from build123d import *

# Parameters (mm, degrees)
SKETCH1_R           = 12.5
SKETCH1_R_2         = 9
BOSS_EXTRUDE1_DEPTH = 10
BOSS_EXTRUDE2_DEPTH = 15
BOSS_EXTRUDE3_DEPTH = 7.5
BOSS_EXTRUDE4_DEPTH = 15
SKETCH3_R           = 3.25
CUT_EXTRUDE1_DEPTH  = 19
SKETCH4_R           = 22.5
CUT_EXTRUDE2_DEPTH  = 151
CUT_EXTRUDE3_DEPTH  = 5


with BuildPart() as part:
    # Sketch1 → Boss-Extrude1 (new body, symmetric)
    with BuildSketch(Plane(origin=(0, 0, 0), x_dir=(0, 0, -1), z_dir=(1, 0, 0))):
        Circle(SKETCH1_R)
        Circle(SKETCH1_R_2, mode=Mode.SUBTRACT)
    extrude(amount=BOSS_EXTRUDE1_DEPTH, both=True)



with BuildPart() as body_2:
    # Sketch1_3 → Boss-Extrude2 (new body, symmetric)
    with BuildSketch(Plane(origin=(0, 0, 0), x_dir=(0, 0, -1), z_dir=(1, 0, 0))):
        with BuildLine():
            Line((22.5, -120.4), (35, -120.4))
            Line((35, -120.4), (35, -117.4))
            Line((35, -117.4), (25.322914524, -117.4))
            ThreePointArc((25.322914524, -117.4), (0, -94.9), (-25.322914524, -117.4))
            Line((-25.322914524, -117.4), (-35, -117.4))
            Line((-35, -117.4), (-35, -120.4))
            Line((-35, -120.4), (-22.5, -120.4))
            ThreePointArc((-22.5, -120.4), (0, -97.9), (22.5, -120.4))
        make_face()
    extrude(amount=BOSS_EXTRUDE2_DEPTH, both=True)


with BuildPart() as part_1:
    add(part.part)

    add(body_2.part)  # Boss-Extrude3 merges body 2
    # Sketch1_7 → Boss-Extrude3 (add, symmetric)
    with BuildSketch(Plane(origin=(0, 0, 0), x_dir=(0, 0, -1), z_dir=(1, 0, 0))):
        with BuildLine():
            ThreePointArc((-15.952867936, -100.506382817), (0, -94.9), (15.952867936, -100.506382817))
            Line((15.952867936, -100.506382817), (8, -9.604686356))
            ThreePointArc((8, -9.604686356), (0, -12.5), (-8, -9.604686356))
            Line((-8, -9.604686356), (-15.952867936, -100.506382817))
        make_face()
    extrude(amount=BOSS_EXTRUDE3_DEPTH, both=True)

    # Sketch2 → Boss-Extrude4 (add)
    with BuildSketch(Plane(origin=(0, -117.4, 0), x_dir=(1, 0, 0), z_dir=(0, 1, 0))):
        with BuildLine():
            Line((-6, 29), (-6, 17))
            Line((-6, 17), (6, 17))
            Line((6, 17), (6, 29))
            ThreePointArc((6, 29), (0, 35), (-6, 29))
        make_face()
    boss_extrude4 = extrude(amount=BOSS_EXTRUDE4_DEPTH)

    # Sketch3 → Cut-Extrude1 (cut, through all)
    with BuildSketch(Plane(origin=(0, -102.4, 0), x_dir=(1, 0, 0), z_dir=(0, 1, 0))):
        with Locations((0, 29)):
            Circle(SKETCH3_R)
    cut_extrude1 = extrude(amount=-CUT_EXTRUDE1_DEPTH, mode=Mode.SUBTRACT)

    # Mirror1: Boss-Extrude4, Cut-Extrude1 across plane
    add(boss_extrude4.mirror(Plane.XY))
    add(cut_extrude1.mirror(Plane.XY), mode=Mode.SUBTRACT)

    # Sketch4 → Cut-Extrude2 (cut)
    with BuildSketch(Plane(origin=(15, 0, 0), x_dir=(0, 0, -1), z_dir=(1, 0, 0))):
        with Locations((0, -120.4)):
            Circle(SKETCH4_R)
    extrude(amount=-CUT_EXTRUDE2_DEPTH, mode=Mode.SUBTRACT)

    # Sketch5 → Cut-Extrude3 (cut)
    with BuildSketch(Plane(origin=(7.5, 0, 0), x_dir=(0, 0, -1), z_dir=(1, 0, 0))):
        with BuildLine():
            ThreePointArc((12.438451255, -94.757556076), (0, -91.9), (-12.438451255, -94.757556076))
            Line((-12.438451255, -94.757556076), (-5.4187458, -14.521955583))
            ThreePointArc((-5.4187458, -14.521955583), (0, -15.5), (5.4187458, -14.521955583))
            Line((5.4187458, -14.521955583), (12.438451255, -94.757556076))
        make_face()
    cut_extrude3 = extrude(amount=-CUT_EXTRUDE3_DEPTH, mode=Mode.SUBTRACT)

    # Mirror2: Cut-Extrude3 across plane
    add(cut_extrude3.mirror(Plane(origin=(0, 0, 0), x_dir=(0, 0, 1), z_dir=(1, 0, 0))), mode=Mode.SUBTRACT)


solid = part_1.part
Geometry check sheet. Reference: the model listing, model coordinates, mm. A direction names the side the tool comes from. Round coordinates to 2 decimals unless told otherwise and drop trailing zeros. Loops run counter-clockwise (first coordinate to the right, second up) from the corner with the lowest first, then second, coordinate; pieces in that order, holes last. Notation, with made-up numbers: (-12.5, -10) - (34.5, -10) arc R19 ccw to (34.5, -6) - close; hole circle Ø2 at (67, -6). An arc over 180 degrees is marked (long way). One line per question, with ' | ' between items. Start each with the question number.
1. Cross-section at C-C on x = 12.75. Record the cut outline in (y, z).
2. Cross-section at B-B on z = 0. Record the cut outline in (x, y).
3. Draft check along Y on faces 1 (the face through (6, -108, -26)), 2 (the face through (-11, -117.4, -30)), 3 (the face through (-5, -91.9, -0.2)), 4 (the face through (7.5, -58, 10)). Enter one of: released by +Y, released by -Y, zero draft, split by the parting line, or undercut.
4. Cross-section at D-D on y = -41. Record the cut outline in (x, z).
5. Depth check by flat-ended pin: pin 1 (3.5 mm diameter, centred on x = -2, z = 29.5, fed in from +Y); pin 2 (16 mm diameter, centred on y = -77, z = 6.5, fed in from -X); pin 3 (14.5 mm diameter, centred on y = 0, z = 0, fed in from +X); pin 4 (12.5 mm diameter, centred on y = -64.5, z = -6, fed in from +X). Enter the tip coordinate at first touch or a pass-through.
6. Scan lines: line 1 (Z direction, x = 0, y = -111); line 2 (X direction, y = -112, z = -29); line 3 (Y direction, x = 2.25, z = 0). Record each from-to range of solid material in increasing order. Write a range as [from, to].
7. Cross-section at A-A on y = 0. Record the cut outline in (x, z).
8. Tool access check on faces 5 (the face through (-5.035, -55.201, 8.978)), 6 (the face through (-6, -108, 26)), 7 (the face through (-10, 3, 9)), 8 (the face through (0.11, -54.42, 11.92)). Record the directions out of +Z, -Z, +X, -X, +Y, -Y that give a thin tool (end or side, any length) a straight path to the whole face; none if there is none.
Taken from the geometry:
1) outline: (-120.4, -35) - (-117.4, -35) - (-117.4, -25.32) arc R25.5 ccw to (-117.4, 25.32) - (-117.4, 35) - (-120.4, 35) - (-120.4, 22.5) arc R22.5 cw to (-120.4, -22.5) - close
2) outline: (-15, -97.9) - (15, -97.9) - (15, -94.9) - (7.5, -94.9) - (7.5, -91.9) - (2.5, -91.9) - (2.5, -15.5) - (7.5, -15.5) - (7.5, -12.5) - (10, -12.5) - (10, -9) - (-10, -9) - (-10, -12.5) - (-7.5, -12.5) - (-7.5, -15.5) - (-2.5, -15.5) - (-2.5, -91.9) - (-7.5, -91.9) - (-7.5, -94.9) - (-15, -94.9) - close; (-10, 9) - (10, 9) - (10, 12.5) - (-10, 12.5) - close
3) face 1: zero draft | face 2: released by +Y | face 3: undercut | face 4: undercut
4) outline: (-7.5, -10.75) - (7.5, -10.75) - (7.5, -7.74) - (2.5, -7.74) - (2.5, 7.74) - (7.5, 7.74) - (7.5, 10.75) - (-7.5, 10.75) - (-7.5, 7.74) - (-2.5, 7.74) - (-2.5, -7.74) - (-7.5, -7.74) - close
5) pin 1: y = -102.4 | pin 2: x = -7.5 | pin 3: through | pin 4: x = 7.5
6) line 1: [-35, -32.25], [-25.75, -20.44], [20.44, 25.75], [32.25, 35] | line 2: [-6, -3.25], [3.25, 6] | line 3: [-97.9, -9], [9, 12.5]
7) outline: (-10, -12.5) - (10, -12.5) - (10, -9) - (-10, -9) - close; (-10, 9) - (10, 9) - (10, 12.5) - (-10, 12.5) - close
8) face 5: -X | face 6: +Z, -X, +Y | face 7: +Z, -Z, -X, +Y | face 8: +Z, +X, -X
